from build123d import *

# Parameters (mm, degrees)
BOSS_EXTRUDE1_DEPTH = 25
BOSS_EXTRUDE2_DEPTH = 5
FILLET1_SIZE        = 3


with BuildPart() as part:
    # Sketch1 → Boss-Extrude1 (new body)
    with BuildSketch(Plane.XY):
        with BuildLine():
            Line((-5, 50), (-52.5, 50))
            Line((-52.5, 50), (-52.5, -50))
            Line((-52.5, -50), (-5, -50))
            Line((-5, -50), (-5, -43.211688234))
            ThreePointArc((-5, -43.211688234), (-43.5, 0), (-5, 43.211688234))
            Line((-5, 43.211688234), (-5, 50))
        make_face()
    extrude(amount=BOSS_EXTRUDE1_DEPTH)

    # Sketch1<3> → Boss-Extrude2 (add)
    with BuildSketch(Plane.XY):
        with BuildLine():
            Line((-5, 29.580398915), (-5, 43.211688234))
            ThreePointArc((-5, 43.211688234), (-43.5, 0), (-5, -43.211688234))
            Line((-5, -43.211688234), (-5, -29.580398915))
            ThreePointArc((-5, -29.580398915), (-30, 0), (-5, 29.580398915))
        make_face()
    extrude(amount=BOSS_EXTRUDE2_DEPTH)

    # Fillet1
    # a fillet whose section is not a circle: 3 mm, written as the material it takes off along each edge
    with BuildSketch(Plane(origin=(-52.5, -50, -7.5), x_dir=(1, 0, 0), z_dir=(0, 0, 1)), Plane(origin=(-52.5, 50, -7.5), x_dir=(0, -1, 0), z_dir=(0, 0, 1)), Plane(origin=(-5, -50, -7.5), x_dir=(0, 1, 0), z_dir=(0, 0, 1))) as fillet1_piece_1:
        with BuildLine():
            Bezier((FILLET1_SIZE, 0), (0, 0), (0, FILLET1_SIZE), weights=[1, 1.222222222, 1])
            Line((0, FILLET1_SIZE), (0, 0))
            Line((0, 0), (FILLET1_SIZE, 0))
        make_face()
    extrude(amount=40, mode=Mode.SUBTRACT)
    with BuildSketch(Plane(origin=(-5, 50, -7.5), x_dir=(0, -1, 0), z_dir=(0, 0, 1))) as fillet1_piece_2:
        with BuildLine():
            Bezier((FILLET1_SIZE, 0), (0, 0), (0, -FILLET1_SIZE), weights=[1, 1.222222222, 1])
            Line((0, -FILLET1_SIZE), (0, 0))
            Line((0, 0), (FILLET1_SIZE, 0))
        make_face()
    extrude(amount=40, mode=Mode.SUBTRACT)
    with BuildSketch(Plane(origin=(-5, 43.211688234, 5), x_dir=(0, 1, 0), z_dir=(0, 0, 1))) as fillet1_piece_3:
        with BuildLine():
            Bezier((2.594970671, 0), (0.073503208, 0), (-0.360297645, 2.483870968), weights=[1, 1.222222222, 1])
            ThreePointArc((-0.360297645, 2.483870968), (-0.162230771, 1.244534585), (0, 0))
            Line((0, 0), (2.594970671, 0))
        make_face()
    extrude(amount=26.487426677, mode=Mode.SUBTRACT)
    with BuildSketch(Plane(origin=(-5, -43.211688234, 5), x_dir=(0, -1, 0), z_dir=(0, 0, 1))) as fillet1_piece_4:
        with BuildLine():
            Bezier((2.594970671, 0), (0.073503208, 0), (-0.360297645, -2.483870968), weights=[1, 1.222222222, 1])
            ThreePointArc((-0.360297645, -2.483870968), (-0.162230771, -1.244534585), (0, 0))
            Line((0, 0), (2.594970671, 0))
        make_face()
    extrude(amount=26.487426677, mode=Mode.SUBTRACT)
    with BuildSketch(Plane(origin=(-5, 29.580398915, -6.088055679), x_dir=(0, 1, 0), z_dir=(0, 0, 1))) as fillet1_piece_5:
        with BuildLine():
            Bezier((2.435222272, 0), (0.092615843, 0), (-0.475288745, 2.272727273), weights=[1, 1.222222222, 1])
            ThreePointArc((-0.475288745, 2.272727273), (-0.215648508, 1.140963567), (0, 0))
            Line((0, 0), (2.435222272, 0))
        make_face()
    extrude(amount=17.176111358, mode=Mode.SUBTRACT)
    with BuildSketch(Plane(origin=(-5, -29.580398915, -6.088055679), x_dir=(0, -1, 0), z_dir=(0, 0, 1))) as fillet1_piece_6:
        with BuildLine():
            Bezier((2.435222272, 0), (0.092615843, 0), (-0.475288745, -2.272727273), weights=[1, 1.222222222, 1])
            ThreePointArc((-0.475288745, -2.272727273), (-0.215648508, -1.140963567), (0, 0))
            Line((0, 0), (2.435222272, 0))
        make_face()
    extrude(amount=17.176111358, mode=Mode.SUBTRACT)


solid = part.part
Build history of the part. All positions in model axes, mm. A direction names the side the tool comes from. Give positions to 0.01 mm unless a question says otherwise; leave off trailing zeros. Loops run counter-clockwise (first coordinate to the right, second up) from the corner with the lowest first, then second, coordinate; pieces in that order, holes last. Notation, with made-up numbers: (65.5, 45.25) - (93.5, 45.25) arc R25 ccw to (93.5, 70.25) - close; hole circle Ø5 at (2.25, -39.75). An arc over 180 degrees is marked (long way). Write item = value, one per line. Start each with the question number.
1) Band-saw the part on D-D on x = -41.5. Give the cut face in (y, z).
2) Drop a flat-ended pin along its axis: pin 1 Ø10 at (x, y) = (-26.5, -1) entering from +Z. Give the stop position or say it passes through.
3) Pull direction Y, two halves, no side cores. Call faces 3 (the cylindrical face through (-43.49, -0.85, 14.86)), 4 (the flat face through (-28, 50, 12)), 5 (the flat face through (-5, 41, 4)): +Y half, -Y half, draft (parallel to the pull), parting line (faces both ways), or undercut.
4) Probe probe 1 along Y at (x, z) = (-40, 16.75); probe 2 along Z at (x, y) = (-17.5, 27); probe 3 along Y at (x, z) = (-18, 22). List the from-to ranges inside material, lowest first. Write a range as from..to.
5) Band-saw the part on A-A on x = -13.5. Give the cut face in (y, z).
6) Band-saw the part on B-B on y = -13.5. Give the cut face in (x, z), plus the area to 3 significant figures.
7) Tool access for faces 1 (the flat face through (-45, 1, 25)), 2 (the flat face through (-33, -1, 5)): list every direction of +Z, -Z, +X, -X, +Y, -Y with a clear straight run to the whole face (end or side of a thin tool).
8) Band-saw the part on C-C on x = -22. Give the cut face in (y, z), plus the area to 3 significant figures.
Final values:
q1.outline = (-50, 0) - (50, 0) - (50, 25) - (13.04, 25) - (13.04, 5) - (-13.04, 5) - (-13.04, 25) - (-50, 25) - close
q2.pin_1 = 5
q3.face_3 = undercut
q3.face_4 = +Y half
q3.face_5 = draft
q4.probe_1 = -50..-17.1, 17.1..50
q4.probe_2 = 0..5
q4.probe_3 = -50..-39.6, 39.6..50
q5.outline = (-50, 0) - (-26.79, 0) - (-26.79, 5) - (-41.35, 5) - (-41.35, 25) - (-50, 25) - close; (26.79, 0) - (50, 0) - (50, 25) - (41.35, 25) - (41.35, 5) - (26.79, 5) - close
q6.outline = (-52.5, 0) - (-26.79, 0) - (-26.79, 5) - (-41.35, 5) - (-41.35, 25) - (-52.5, 25) - close
q6.area = 352 mm²
q7.face_1 = +Z, +X, -X, +Y, -Y
q7.face_2 = +Z, +X
q8.outline = (-50, 0) - (-20.4, 0) - (-20.4, 5) - (-37.53, 5) - (-37.53, 25) - (-50, 25) - close; (20.4, 0) - (50, 0) - (50, 25) - (37.53, 25) - (37.53, 5) - (20.4, 5) - close
q8.area = 795 mm²
